Model file for the job. Use its own axes, mm. A direction names the side the tool comes from. Round coordinates to 2 decimals unless told otherwise and drop trailing zeros. Order: outer loops, then holes, each group sorted by start corner. A loop starts at its lowest first (then second) coordinate and runs counter-clockwise, first axis right, second up. Notation, with made-up numbers: (66, 42) -> (110, 42) arc R21 cw to (110, 76) -> close; hole circle Ø10 at (-35, 73). An arc over 180 degrees is marked (long way). Use CSV: the item, a comma, the result in double quotes.
Autodesk Inventor part; units mm, degrees
ref_plane "YZ Plane" through (0, 0, 0) normal (1, 0, 0) x (0, 1, 0)
ref_plane "XZ Plane" through (0, 0, 0) normal (0, 1, 0) x (-1, 0, 0)
ref_plane "XY Plane" through (0, 0, 0) normal (0, 0, 1) x (1, 0, 0)
sketch "Sketch1" plane through (0, 0, 0) normal (1, 0, 0) x (0, 1, 0)
  line L0 (0, 0) -> (9.779, 0)
  line L1 (9.779, 0) -> (9.779, -77.47)
  line L2 (9.779, -77.47) -> (0, -77.47)
  line L3 (0, -77.47) -> (0, 0)
  line L4 (3.175, -3.175) -> (6.604, -3.175)
  line L5 (6.604, -3.175) -> (6.604, -74.295)
  line L6 (6.604, -74.295) -> (3.175, -74.295)
  line L7 (3.175, -74.295) -> (3.175, -3.175)
  dimension "d0" = 3.175
  dimension "d1" = 3.175
  dimension "d2" = 3.175
  dimension "d3" = 3.175
  dimension "d4" = 3.429
  dimension "d5" = 71.12
extrude "Extrusion1" add sketch "Sketch1" along normal blind 104.902
sketch "Sketch2" plane through (0, 0, 0) normal (-1, 0, 0) x (0, 0, 1)
  line L0 (-77.47, 0) -> (-77.47, 9.779)
  line L1 (0, 9.779) -> (0, 0)
  line L2 (-77.47, 9.779) -> (0, 9.779)
  line L3 (0, 9.779) -> (0, 0)
  line L4 (0, 0) -> (-77.47, 0)
  line L5 (-77.47, 0) -> (-77.47, 9.779)
extrude "Extrusion2" add sketch "Sketch2" along normal blind 3.175
sketch "Sketch3" plane through (104.902, 0, 0) normal (1, 0, 0) x (0, 0, -1)
  line L0 (0, 0) -> (77.47, 0)
  line L1 (69.5325, 6.604) -> (2.8575, 6.604)
  line L2 (2.8575, 6.604) -> (2.8575, 0)
  line L3 (2.8575, 0) -> (69.5325, 0)
  line L4 (69.5325, 0) -> (69.5325, 6.604)
  line L5 (77.47, 0) -> (77.47, 9.779)
  dimension "d10" = 7.9375
  dimension "d11" = 66.675
extrude "Extrusion3" cut sketch "Sketch3" against normal blind 3.175
properties part number "HardDriveCase"
Q1. Which spindle directions (+Z, -Z, +X, -X, +Y, -Y) get a long thin tool onto all of the face, cutting with end or side? Do faces 1 (the flat face through (52, 3.175, -39)), 2 (the flat face through (101.727, 2, -36)), 3 (the flat face through (50, 5, 0)). Say none if no direction does.
From the geometry:
face 1,"+X"
face 2,"+X, -Y"
face 3,"+Z, +X, -X, +Y, -Y"
Q2. Cut at D-D (z = -57.5). Give the cut face in (x, y) (3 decimals), plus the area to 3 significant figures.
From the geometry:
outline,"(-3.175, 0) -> (101.727, 0) -> (101.727, 3.175) -> (0, 3.175) -> (0, 6.604) -> (104.902, 6.604) -> (104.902, 9.779) -> (-3.175, 9.779) -> close"
area,"687 mm²"
Q3. Probe line 1 along Y through (x, z) = (8, -68) (3 decimals); line 2 along Z through (x, y) = (73, 4.75) (3 decimals); line 3 along X through (y, z) = (2.25, -15.5) (3 decimals). List the from-to ranges inside material, lowest first.
From the geometry:
line 1,"y = 0 to 3.175, 6.604 to 9.779"
line 2,"z = -77.47 to -74.295, -3.175 to 0"
line 3,"x = -3.175 to 101.727"
Q4. Cut at A-A (x = 14). Give the cut face in (y, z) (3 decimals), plus the area to 3 significant figures.
From the geometry:
outline,"(0, -77.47) -> (9.779, -77.47) -> (9.779, 0) -> (0, 0) -> close; hole (3.175, -74.295) -> (6.604, -74.295) -> (6.604, -3.175) -> (3.175, -3.175) -> close"
area,"514 mm²"
Q5. Mould opens along Y. For faces 4 (the flat face through (50, 9.779, -38)), 5 (the flat face through (50, 5, -3.175)), 6 (the flat face through (50, 5, -77.47)) say: +Y half, -Y half, draft (parallel to the pull), parting line (faces both ways), or undercut.
From the geometry:
face 4,"+Y half"
face 5,"undercut"
face 6,"draft"
Q6. Cut at B-B (z = -72). Give the cut face in (x, y) (3 decimals), plus the area to 3 significant figures.
From the geometry:
outline,"(-3.175, 0) -> (104.902, 0) -> (104.902, 3.175) -> (0, 3.175) -> (0, 6.604) -> (104.902, 6.604) -> (104.902, 9.779) -> (-3.175, 9.779) -> close"
area,"697 mm²"
Q7. Pin check, flat tips, straight feed: pin 1 (1 mm diameter, centred on y = 5, z = -31.5, fed in from +X); pin 2 (2 mm diameter, centred on y = 3, z = -27.5, fed in from +X). Stop position of each tip, or through.
From the geometry:
pin 1,"stops at x = 0"
pin 2,"stops at x = 101.73"
